Design review of the part shown in the three views and the two pictorial views. Dimensions are in mm from the part's minimum x, y and z. A direction names the side the tool comes from. Give positions to 0.01 mm unless a question says otherwise; leave off trailing zeros. Write each loop counter-clockwise with the first axis right and the second up, starting at its lowest first coordinate (ties: lowest second). Pieces come first, ordered by that corner, then holes.
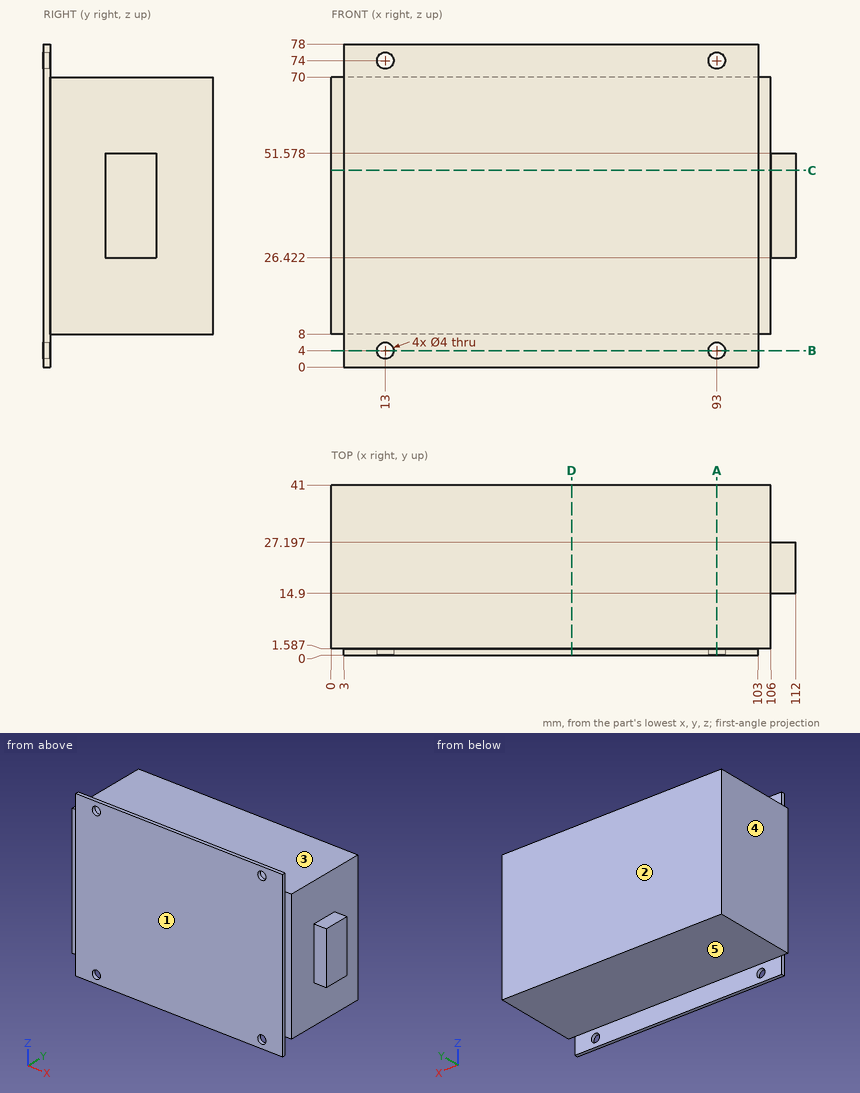
(1) Consider section D-D, the plane x = 58. Give the boundary of the cut face in (y, z).
Resolved:
outline: (0, 0) - (1.59, 0) - (1.59, 8) - (41, 8) - (41, 70) - (1.59, 70) - (1.59, 78) - (0, 78) - close
(2) To check wall thickness, follow L1, parallel to X at y = 1.15, z = 74; L2, parallel to Z at x = 52.5, y = 21; L3, parallel to X at y = 7.5, z = 37. State the ranges of each line that lie inside material, in increasing order.
Resolved:
L1: x = 3 to 11, 15 to 91, 95 to 103
L2: z = 8 to 70
L3: x = 0 to 106
(3) Consider section A-A, the plane x = 93. Give the boundary of the cut face in (y, z).
Resolved:
outline: (0, 0) - (1.59, 0) - (1.59, 2) - (0, 2) - close; (0, 6) - (1.59, 6) - (1.59, 8) - (41, 8) - (41, 70) - (1.59, 70) - (1.59, 72) - (0, 72) - close; (0, 76) - (1.59, 76) - (1.59, 78) - (0, 78) - close
(4) Clearance check with flat-ended pins moving along their axes: P1, Ø6.5, axis at x = 64.5, z = 75.5, coming from the +Y side; P2, Ø6, axis at y = 28, z = 63, coming from the +X side; P3, Ø5, axis at x = 109.5, y = 19, coming from the -Z side; P4, Ø6.5, axis at x = 13, z = 74, coming from the -Y side. State where each tip first meets the part, or that it passes through.
Resolved:
P1: stops at y = 1.59
P2: stops at x = 106
P3: stops at z = 26.42
P4: stops at y = 0
(5) Tool access review of the marked faces 4 and 5: name each direction out of +Z, -Z, +X, -X, +Y, -Y from which nothing blocks a thin tool from reaching the whole face with its end or side.
Resolved:
face 4: +Z, -Z, -X, +Y, -Y
face 5: -Z, +X, -X, +Y
(6) Consider section B-B, the plane z = 4. Give the boundary of the cut face in (x, y), then the cut area to 3 significant figures.
Resolved:
outline: (3, 0) - (11, 0) - (11, 1.59) - (3, 1.59) - close; (15, 0) - (91, 0) - (91, 1.59) - (15, 1.59) - close; (95, 0) - (103, 0) - (103, 1.59) - (95, 1.59) - close
area: 146 mm2
(7) Consider section C-C, the plane z = 47.5. Give the boundary of the cut face in (x, y), then the cut area to 3 significant figures.
Resolved:
outline: (0, 1.59) - (3, 1.59) - (3, 0) - (103, 0) - (103, 1.59) - (106, 1.59) - (106, 14.9) - (112, 14.9) - (112, 27.2) - (106, 27.2) - (106, 41) - (0, 41) - close
area: 4,410 mm2
(8) Mouldability with a two-part tool opening along Y and no side actions: class the marked faces 1, 2 and 3 as pulls with the +Y half, pulls with the -Y half, needs draft (parallel to the pull), parting line crosses it, or undercut.
Resolved:
face 1: pulls with the -Y half
face 2: pulls with the +Y half
face 3: needs draft
